```python
from build123d import *

# Parameters (mm, degrees)
SKETCH1_W           = 34
SKETCH1_H           = 46.5
BOSS_EXTRUDE1_DEPTH = 28.5
SKETCH2_R           = 10.25
BOSS_EXTRUDE2_DEPTH = 2
SKETCH3_R           = 4
BOSS_EXTRUDE3_DEPTH = 1.9
SKETCH10_R          = 1.126890163
CUT_EXTRUDE2_DEPTH  = 4


with BuildPart() as part:
    # Sketch1 → Boss-Extrude1 (new body)
    with BuildSketch(Plane.XY):
        Rectangle(SKETCH1_W, SKETCH1_H)
    extrude(amount=BOSS_EXTRUDE1_DEPTH)

    # Sketch2 → Boss-Extrude2 (add)
    with BuildSketch(Plane(origin=(17, 0, 0), x_dir=(0, 0, -1), z_dir=(1, 0, 0))):
        with Locations((-14.25, 12)):
            Circle(SKETCH2_R)
    extrude(amount=BOSS_EXTRUDE2_DEPTH)

    # Sketch3 → Boss-Extrude3 (add)
    with BuildSketch(Plane(origin=(19, 0, 0), x_dir=(0, 0, -1), z_dir=(1, 0, 0))):
        with Locations(Location((-14.25, 12, 0), (0, 0, 180))):
            Circle(SKETCH3_R)
    extrude(amount=BOSS_EXTRUDE3_DEPTH)

    # Sketch10 → Cut-Extrude2 (cut)
    with BuildSketch(Plane(origin=(17, 0, 0), x_dir=(0, 0, -1), z_dir=(1, 0, 0))):
        with Locations((-3.25, 20)):
            Circle(SKETCH10_R)
        with Locations((-25.25, 20)):
            Circle(SKETCH10_R)
        with Locations((-25.25, -20)):
            Circle(SKETCH10_R)
        with Locations((-3.25, -20)):
            Circle(SKETCH10_R)
    cut_extrude2 = extrude(amount=-CUT_EXTRUDE2_DEPTH, mode=Mode.SUBTRACT)

    # Mirror1: Cut-Extrude2 across plane
    add(cut_extrude2.mirror(Plane(origin=(0, 0, 0), x_dir=(0, 0, 1), z_dir=(1, 0, 0))), mode=Mode.SUBTRACT)


solid = part.part
```
Input: part model. Units: mm. Frame: model coordinates. A direction names the side the tool comes from. Coordinates: 2 decimals unless noted, no trailing zeros. Loops run counter-clockwise (first coordinate to the right, second up) from the corner with the lowest first, then second, coordinate; pieces in that order, holes last.
Q1. Set-up query: faces 1 (the flat face through (0, -23.25, 14)), 2 (the cylindrical face through (15.028, 20.05, 26.376)), 3 (the cylindrical face through (-15.028, 20.05, 26.376)). Return all of +Z, -Z, +X, -X, +Y, -Y with unobstructed straight access to the full face (end or side cutting, diameter ignored); none if empty.
Results are:
face 1: +Z, -Z, +X, -X, -Y
face 2: +X
face 3: -X
Q2. Line query: line 1 along Y through (x, z) = (16.05, 25.25); line 2 along X through (y, z) = (20, 20.5); line 3 along X through (y, z) = (-12, 20.75). Output: solid intervals per line, ascending.
Results are:
line 1: y = -23.25 to -21.13, -18.87 to 18.87, 21.13 to 23.25
line 2: x = -17 to 19
line 3: x = -17 to 17
Q3. Section A-A, the plane z = 14.25. Return the cut outline in (x, y), and give its area (3 significant figures).
Results are:
outline: (-17, -23.25) - (17, -23.25) - (17, 1.75) - (19, 1.75) - (19, 8) - (20.9, 8) - (20.9, 16) - (19, 16) - (19, 22.25) - (17, 22.25) - (17, 23.25) - (-17, 23.25) - close
area: 1,640 mm2
Q4. Mould query, pull axis Y, two halves, no side actions, for faces 4 (the flat face through (13, 20, 3)), 5 (the flat face through (0, 0, 28.5)), 6 (the flat face through (0, 23.25, 14)). Classes: +Y half, -Y half, draft (parallel to the pull), parting line (faces both ways), or undercut.
Results are:
face 4: undercut
face 5: draft
face 6: +Y half
Q5. Section D-D, the plane y = 4.5. Return the cut outline in (x, z).
Results are:
outline: (-17, 0) - (17, 0) - (17, 7.26) - (19, 7.26) - (19, 21.24) - (17, 21.24) - (17, 28.5) - (-17, 28.5) - close
Q6. Section C-C, the plane z = 3.25. Return the cut outline in (x, y), and give its area (3 significant figures).
Results are:
outline: (-17, -23.25) - (17, -23.25) - (17, -21.13) - (13, -21.13) - (13, -18.87) - (17, -18.87) - (17, 18.87) - (13, 18.87) - (13, 21.13) - (17, 21.13) - (17, 23.25) - (-17, 23.25) - (-17, 21.13) - (-13, 21.13) - (-13, 18.87) - (-17, 18.87) - (-17, -18.87) - (-13, -18.87) - (-13, -21.13) - (-17, -21.13) - close
area: 1,540 mm2
Q7. Section B-B, the plane y = 12. Return the cut outline in (x, z), and give its area (3 significant figures).
Results are:
outline: (-17, 0) - (17, 0) - (17, 4) - (19, 4) - (19, 10.25) - (20.9, 10.25) - (20.9, 18.25) - (19, 18.25) - (19, 24.5) - (17, 24.5) - (17, 28.5) - (-17, 28.5) - close
area: 1,030 mm2
Q8. Contact query for flat-ended pins moving along their axis: pin 1 (5 mm diameter, centred on y = -12.5, z = 12, fed in from +X); pin 2 (2 mm diameter, centred on y = 20, z = 3.25, fed in from -X); pin 3 (2 mm diameter, centred on y = -20, z = 3.25, fed in from +X). Output: stop coordinate, or through.
Results are:
pin 1: stops at x = 17
pin 2: stops at x = -13
pin 3: stops at x = 13
